from build123d import *

# Parameters (mm, degrees)
M2_5X0_45_TAPPED_HOLE2_D     = 2.05
M2_5X0_45_TAPPED_HOLE2_DEPTH = 6.35
M2_5X0_45_TAPPED_HOLE2_TIP   = 0.615882135
CUT_EXTRUDE1_DEPTH           = 56.113519213


with BuildPart() as part:
    # Sketch1 → Revolve1 (revolve)
    with BuildSketch(Plane.XY, mode=Mode.PRIVATE) as revolve1_sk:
        Polygon((-15, 27.5), (0, 27.5), (0, 37.5), (-2, 37.5), (-2, 29.5), (-12, 29.5), (-12, 37.5), (-15, 37.5), align=None)
    revolve(revolve1_sk.sketch.rotate(Axis((0, 0, 0), (-1, 0, 0)), 90), axis=Axis((0, 0, 0), (-1, 0, 0)))

    # M2.5x0.45 Tapped Hole2
    with Locations(Plane.ZY.offset(15)):
        with Locations((0, -32.5), (-32.5, 0), (32.5, 0), (0, 32.5)):
            Hole(M2_5X0_45_TAPPED_HOLE2_D / 2, depth=M2_5X0_45_TAPPED_HOLE2_DEPTH)
            with Locations((0, 0, -(M2_5X0_45_TAPPED_HOLE2_DEPTH + M2_5X0_45_TAPPED_HOLE2_TIP / 2))):  # 118° drill point
                Cone(0, M2_5X0_45_TAPPED_HOLE2_D / 2, M2_5X0_45_TAPPED_HOLE2_TIP, mode=Mode.SUBTRACT)

    # Sketch6 → Cut-Extrude1 (cut, through all)
    with BuildSketch(Plane(origin=(0, 0, 0), x_dir=(0, 0, -1), z_dir=(1, 0, 0))):
        Polygon((27.223611076, -25.809397513), (25.809397513, -27.223611076), (18.725468962, -20.139682524), (20.139682524, -18.725468962), align=None)
    extrude(amount=-CUT_EXTRUDE1_DEPTH, mode=Mode.SUBTRACT)


solid = part.part
Source: CAD feature listing. Evaluate the final solid. Frame: model axes, mm. A direction names the side the tool comes from. Give positions to 0.01 mm unless a question says otherwise; leave off trailing zeros. Write each loop counter-clockwise with the first axis right and the second up, starting at its lowest first coordinate (ties: lowest second). Pieces come first, ordered by that corner, then holes. Notation, with made-up numbers: M 88,4 L 97,4 A27 ccw 97,36 Z; hole C 19.25,-19 d11. An arc over 180 degrees is marked long. Return JSON: item names as keys, results as strings. Group by question number.
1) Set-up query: faces 3 (the face through (-9.062, -21.368, -19.954)), 4 (the face through (-2, -22, 20)), 5 (the face through (-13.479, -31.484, 0.133)), 6 (the face through (-15, 28, -3)). Return all of +Z, -Z, +X, -X, +Y, -Y with unobstructed straight access to the full face (end or side cutting, diameter ignored); none if empty.
2) Cut plane C-C, the plane z = 15. Output: boundary loops of the cut face in (x, y), plus the area to 3 significant figures.
3) Material intervals for line 1 along X through (y, z) = (31.5, 9.5); line 2 along Y through (x, z) = (-6.25, 0); line 3 along Z through (x, y) = (-5.25, -23), sorted ascending. Write a range as [from, to].
4) Cut plane A-A, the plane z = 0. Output: boundary loops of the cut face in (x, y) (3 decimals), plus the area to 3 significant figures.
5) Pull-direction query (Z, two-part tool) for faces 1 (the face through (0, 3, 28)), 2 (the face through (-9.062, -19.855, -21.269)); classes: pulls with the +Z half, pulls with the -Z half, needs draft (parallel to the pull), parting line crosses it, or undercut.
6) Cut plane B-B, the plane y = 32.5. Output: boundary loops of the cut face in (x, z) (3 decimals).
7) Cut plane D-D, the plane y = -9. Output: boundary loops of the cut face in (x, z), plus the area to 3 significant figures.
8) Pin query (flat end, axial travel): P1, Ø8, axis at x = -8.5, z = 6.5, coming from the +Y side; P2, Ø3, axis at x = -6, y = -6, coming from the -Z side; P3, Ø6, axis at x = -3, z = 13, coming from the +Y side; P4, Ø8, axis at y = -27.5, z = -2.5, coming from the +X side. Return the tip coordinate at first contact, or that it passes through.
Recorded:
{
 "1": {"face 3": "+X, -X", "face 4": "none", "face 5": "-X", "face 6": "+Z, -Z, -X, +Y, -Y"},
 "2": {"outline": "M -15,-34.37 L -12,-34.37 L -12,-25.4 L -2,-25.4 L -2,-34.37 L 0,-34.37 L 0,-23.05 L -15,-23.05 Z; M -15,23.05 L 0,23.05 L 0,34.37 L -2,34.37 L -2,25.4 L -12,25.4 L -12,34.37 L -15,34.37 Z", "area": "160 mm²"},
 "3": {"line 1": "x = [-15, -12], [-2, 0]", "line 2": "y = [-29.5, -27.5], [27.5, 29.5]", "line 3": "z = [-18.47, -15.07], [15.07, 18.47]"},
 "4": {"outline": "M -15,-37.5 L -12,-37.5 L -12,-33.525 L -15,-33.525 Z; M -15,-31.475 L -12,-31.475 L -12,-29.5 L -2,-29.5 L -2,-37.5 L 0,-37.5 L 0,-27.5 L -15,-27.5 Z; M -15,27.5 L 0,27.5 L 0,37.5 L -2,37.5 L -2,29.5 L -12,29.5 L -12,31.475 L -15,31.475 Z; M -15,33.525 L -12,33.525 L -12,37.5 L -15,37.5 Z", "area": "128 mm²"},
 "5": {"face 1": "needs draft", "face 2": "undercut"},
 "6": {"outline": "M -15,-18.708 L -12,-18.708 L -12,-1.025 L -15,-1.025 Z; M -15,1.025 L -12,1.025 L -12,18.708 L -15,18.708 Z; M -2,-18.708 L 0,-18.708 L 0,18.708 L -2,18.708 Z"},
 "7": {"outline": "M -15,-36.4 L -12,-36.4 L -12,-28.09 L -2,-28.09 L -2,-36.4 L 0,-36.4 L 0,-25.99 L -15,-25.99 Z; M -15,25.99 L 0,25.99 L 0,36.4 L -2,36.4 L -2,28.09 L -12,28.09 L -12,36.4 L -15,36.4 Z", "area": "146 mm²"},
 "8": {"P1": "stops at y = 37.22", "P2": "stops at z = -29.15", "P3": "stops at y = 36.09", "P4": "stops at x = 0"}
}
